Build history of the part. All positions in model axes, mm. Face numbers are marked on the shaded views. A direction names the side the tool comes from. Give positions to 0.01 mm unless a question says otherwise; leave off trailing zeros. Write each loop counter-clockwise with the first axis right and the second up, starting at its lowest first coordinate (ties: lowest second). Pieces come first, ordered by that corner, then holes. Notation, with made-up numbers: (4, 34) -> (30, 34) arc R28 ccw to (30, 69) -> close; hole circle Ø11 at (0, -22.5). An arc over 180 degrees is marked (long way). Put each result on its own line as item: value.
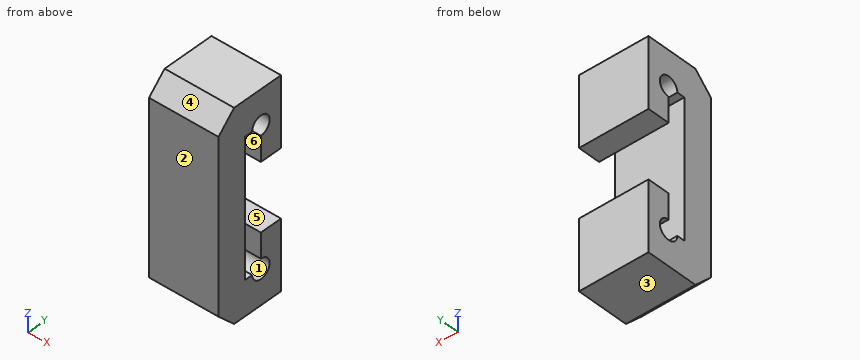
Autodesk Inventor part; units mm, degrees
ref_plane "YZ Plane" through (0, 0, 0) normal (1, 0, 0) x (0, 1, 0)
ref_plane "XZ Plane" through (0, 0, 0) normal (0, 1, 0) x (-1, 0, 0)
ref_plane "XY Plane" through (0, 0, 0) normal (0, 0, 1) x (1, 0, 0)
sketch "Sketch1" plane through (0, 0, 0) normal (1, 0, 0) x (0, 1, 0)
  arc A0 (0, 16.1546) -> (-0.889, 17.0436) centre (0, 17.0436) ccw
  arc A1 (-0.889, 4.5468) -> (0, 5.4358) centre (0, 4.5468) ccw
  line L0 (0, 13.8686) -> (2.0409, 13.8686)
  line L1 (0, 7.7218) -> (2.0409, 7.7218)
  line L2 (2.0409, 7.7218) -> (2.0409, 1.3718)
  line L3 (2.0409, 1.3718) -> (-2.7216, 1.3718)
  line L4 (2.0409, 13.8686) -> (2.0409, 20.2186)
  line L5 (2.0409, 20.2186) -> (-2.7216, 20.2186)
  line L6 (-4.3091, 18.6311) -> (-4.3091, 2.9593)
  line L7 (-2.7216, 20.2186) -> (-4.3091, 18.6311)
  line L8 (-2.7216, 1.3718) -> (-4.3091, 2.9593)
  line L9 (0, 3.6578) -> (-1.5964, 3.6578)
  line L10 (-1.5964, 4.5468) -> (-1.5964, 17.0436)
  line L11 (-1.5964, 17.9326) -> (0, 17.9326)
  line L12 (0, 16.1546) -> (0, 13.8686)
  line L13 (0, 7.7218) -> (0, 5.4358)
  line L14 (-0.889, 4.5468) -> (-1.5964, 4.5468)
  line L15 (-0.889, 17.0436) -> (-1.5964, 17.0436)
  point P0 (0, 0)
  point P1 (-4.3091, 1.3718)
  point P2 (-4.3091, 20.2186)
  dimension "d0" = 14.2748
  dimension "d1" = 1.778
  dimension "d2" = 0.889
  dimension "d3" = 1.778
  dimension "d4" = 0.889
  dimension "d5" = 3.175
  dimension "d6" = 3.175
  dimension "d7" = 6.35
  dimension "d8" = 6.35
  dimension "d9" = 6.35
  dimension "d10" = 1.5875
  dimension "d11" = 1.5875
  dimension "d12" = 1.5875
  dimension "d13" = 1.5875
extrude "Extrusion1" add sketch "Sketch1" along normal blind 6.35
properties part number "led_clip_v2"
1) Slice it at B-B (y = 1.5). Write the cut outline in (x, z).
Filled sheet:
outline: (0, 1.37) -> (6.35, 1.37) -> (6.35, 7.72) -> (0, 7.72) -> close; (0, 13.87) -> (6.35, 13.87) -> (6.35, 20.22) -> (0, 20.22) -> close
2) Wall check: L1, parallel to Y at x = 4, z = 15; L2, parallel to Z at x = 2.5, y = 1.75; L3, parallel to Z at x = 1.75, y = -1.25. Give the ranges that are in metal, low to high.
Filled sheet:
L1: -4.31 to -1.6, 0 to 2.04
L2: 1.37 to 7.72, 13.87 to 20.22
L3: 1.37 to 4.55, 17.04 to 20.22
3) Slice it at A-A (z = 15.25). Write the cut outline in (x, y).
Filled sheet:
outline: (0, -4.31) -> (6.35, -4.31) -> (6.35, -1.6) -> (0, -1.6) -> close; (0, 0) -> (6.35, 0) -> (6.35, 2.04) -> (0, 2.04) -> close
4) Slice it at C-C (x = 3.75). Write the cut outline in (y, z).
Filled sheet:
outline: (-4.31, 2.96) -> (-2.72, 1.37) -> (2.04, 1.37) -> (2.04, 7.72) -> (0, 7.72) -> (0, 5.44) arc R0.89 cw (long way) to (-0.89, 4.55) -> (-1.6, 4.55) -> (-1.6, 17.04) -> (-0.89, 17.04) arc R0.89 cw (long way) to (0, 16.15) -> (0, 13.87) -> (2.04, 13.87) -> (2.04, 20.22) -> (-2.72, 20.22) -> (-4.31, 18.63) -> close
5) Tool access for the marked faces 4, 5 and 6: list every direction of +Z, -Z, +X, -X, +Y, -Y with a clear straight run to the whole face (end or side of a thin tool).
Filled sheet:
face 4: +Z, +X, -X, -Y
face 5: +X, -X, +Y
face 6: +X, -X
6) Slice it at D-D (z = 11.5). Write the cut outline in (x, y).
Filled sheet:
outline: (0, -4.31) -> (6.35, -4.31) -> (6.35, -1.6) -> (0, -1.6) -> close
7) Pull direction Y, two halves, no side cores. Call the marked faces 1, 2 and 3: released by +Y, released by -Y, zero draft, split by the parting line, or undercut.
Filled sheet:
face 1: undercut
face 2: released by -Y
face 3: zero draft
8) Pin check, flat tips, straight feed: pin 1 (3 mm diameter, centred on y = 0, z = 4, fed in from +X); pin 2 (1.1 mm diameter, centred on y = 0, z = 17.04, fed in from +X). Stop position of each tip, or through.
Filled sheet:
pin 1: x = 6.35
pin 2: through
